Build history of the part. All positions in model axes, mm. Face numbers are marked on the shaded views. A direction names the side the tool comes from. Give positions to 0.01 mm unless a question says otherwise; leave off trailing zeros. Order: outer loops, then holes, each group sorted by start corner. A loop starts at its lowest first (then second) coordinate and runs counter-clockwise, first axis right, second up. Notation, with made-up numbers: (36, -40) - (47, -40) arc R4 cw to (47, -33) - close; hole circle Ø10 at (-27.75, -33). An arc over 180 degrees is marked (long way). Answer in a Markdown table with one row per item.
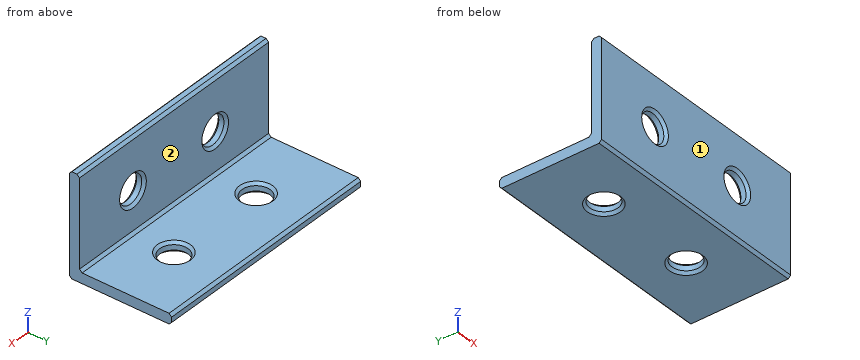
```python
from build123d import *

# Parameters (mm, degrees)
F1_DEPTH  = 50
F2_SIZE   = 0.5
F3_R      = 2.75
F4_DEPTH  = 25
F5_SIZE   = 0.5
F6_R      = 2.75
F7_DEPTH  = 25
F8_SIZE   = 0.5
F9_W      = 1.5
F9_H      = 19
F10_DEPTH = 25


with BuildPart() as f1:
    # F0 (on Right) → F1 (new body)
    with BuildSketch(Plane.YZ):
        Polygon((18, 0), (0, 0), (0, 18), (-2, 18), (-2, -2), (18, -2), align=None)
    extrude(amount=F1_DEPTH)

    # F2
    f2_edges = [f1.edges().sort_by_distance(p)[0] for p in [
        (25, 0, 18),
        (25, -2, 18),
        (0, -1, 18),
        (50, -1, 18),
        (25, 18, 0),
        (25, 0, 0),
        (0, 9, 0),
        (50, 9, 0),
        (25, -2, -2),
        (25, 18, -2),
        (0, 8, -2),
        (50, 8, -2),
        (0, -2, 8),
        (50, -2, 8),
    ]]
    chamfer(f2_edges, length=F2_SIZE)

    # F3 (on face) → F4 (cut)
    with BuildSketch(Plane(origin=(0, 0, 0), x_dir=(-1, 0, 0), z_dir=(0, 1, 0))):
        with Locations((-15, 8)):
            Circle(F3_R)
        with Locations((-35, 8)):
            Circle(F3_R)
    extrude(amount=-F4_DEPTH, mode=Mode.SUBTRACT)

    # F5
    f5_edges = [f1.edges().sort_by_distance(p)[0] for p in [
        (17.75, 0, 8),
        (12.25, -1, 8),
        (17.75, -2, 8),
        (37.75, 0, 8),
        (32.25, -1, 8),
        (37.75, -2, 8),
    ]]
    chamfer(f5_edges, length=F5_SIZE)

    # F6 (on face) → F7 (cut)
    with BuildSketch(Plane(origin=(0, 0, -2), x_dir=(1, 0, 0), z_dir=(0, 0, -1))):
        with Locations((15, -8)):
            Circle(F6_R)
        with Locations((35, -8)):
            Circle(F6_R)
    extrude(amount=-F7_DEPTH, mode=Mode.SUBTRACT)

    # F8
    f8_edges = [f1.edges().sort_by_distance(p)[0] for p in [
        (12.25, 8, -2),
        (17.75, 8, -1),
        (12.25, 8, 0),
        (32.25, 8, -2),
        (37.75, 8, -1),
        (32.25, 8, 0),
    ]]
    chamfer(f8_edges, length=F8_SIZE)

    # F9 (on face) → F10 (cut)
    with BuildSketch(Plane.XZ.offset(2)):
        Polygon((51.7472885549, 18), (48, 18), (48, 17.5), (49.5, 17.5), (49.5, -1.5), (48, -1.5), (48, -2), (48, -2.0400607027), (51.7472885549, -2.0400607027), align=None)
        with Locations((48.75, 8)):
            Rectangle(F9_W, F9_H)
        Polygon((2, 17.5), (2, 18), (2, 19.6672808379), (-2.285732422, 19.6672808379), (-2.285732422, -2), (2, -2), (2, -1.5), (0.5, -1.5), (0.5, 17.5), align=None)
        with Locations((1.25, 8)):
            Rectangle(F9_W, F9_H)
    extrude(amount=-F10_DEPTH, mode=Mode.SUBTRACT)


solid = f1.part
```
1. Cut at D-D on x = 8. Write the cut outline in (y, z), and give its area (3 significant figures).
Check result:
| item | result |
|---|---|
| outline | (-2, -1.5) - (-1.5, -2) - (17.5, -2) - (18, -1.5) - (18, -0.5) - (17.5, 0) - (0.5, 0) - (0, 0.5) - (0, 17.5) - (-0.5, 18) - (-1.5, 18) - (-2, 17.5) - close |
| area | 75.5 mm² |
2. Cut at C-C on x = 15. Write the cut outline in (y, z).
Check result:
| item | result |
|---|---|
| outline | (-2, -1.5) - (-1.5, -2) - (4.75, -2) - (5.25, -1.5) - (5.25, -0.5) - (4.75, 0) - (0.5, 0) - (0, 0.5) - (0, 4.75) - (-0.5, 5.25) - (-1.5, 5.25) - (-2, 4.75) - close; (-2, 11.25) - (-1.5, 10.75) - (-0.5, 10.75) - (0, 11.25) - (0, 17.5) - (-0.5, 18) - (-1.5, 18) - (-2, 17.5) - close; (10.75, -1.5) - (11.25, -2) - (17.5, -2) - (18, -1.5) - (18, -0.5) - (17.5, 0) - (11.25, 0) - (10.75, -0.5) - close |
3. Which spindle directions (+Z, -Z, +X, -X, +Y, -Y) get a long thin tool onto all of the face, cutting with end or side? Do the marked faces 1 and 2. Say none if no direction does.
Check result:
| item | result |
|---|---|
| face 1 | +Z, -Z, +X, -X, -Y |
| face 2 | +Z, +X, -X, +Y |
4. Cut at A-A on z = 8. Write the cut outline in (x, y), and give its area (3 significant figures).
Check result:
| item | result |
|---|---|
| outline | (2, -2) - (11.75, -2) - (12.25, -1.5) - (12.25, -0.5) - (11.75, 0) - (2, 0) - close; (17.75, -1.5) - (18.25, -2) - (31.75, -2) - (32.25, -1.5) - (32.25, -0.5) - (31.75, 0) - (18.25, 0) - (17.75, -0.5) - close; (37.75, -1.5) - (38.25, -2) - (48, -2) - (48, 0) - (38.25, 0) - (37.75, -0.5) - close |
| area | 69.0 mm² |
5. Probe line 1 (Z direction, x = 35, y = -0.8); line 2 (X direction, y = 8, z = -1.2); line 3 (X direction, y = -0.5, z = 6.25). List the from-to ranges inside material, lowest first.
Check result:
| item | result |
|---|---|
| line 1 | z = -2 to 5.25, 10.75 to 18 |
| line 2 | x = 2 to 12.25, 17.75 to 32.25, 37.75 to 48 |
| line 3 | x = 2 to 12.88, 17.12 to 32.88, 37.12 to 48 |
6. Drop flat-ended pins along their axis: P1, Ø4, axis at x = 35.5, y = 12.5, coming from the +Z side; P2, Ø2, axis at x = 13, y = 8.5, coming from the +Z side; P3, Ø7, axis at x = 15, z = 8, coming from the +Y side. Give the stop position or say it passes through.
Check result:
| item | result |
|---|---|
| P1 | stops at z = 0 |
| P2 | stops at z = -0.19 |
| P3 | stops at y = 0 |
